```python
from build123d import *

# Parameters (mm, degrees)
F0_R     = 25
F1_DEPTH = 75
F0_R_2   = 37.5
F2_DEPTH = 50
F3_R     = 18
F4_DEPTH = 37.501
F5_R     = 25
F6_DEPTH = 37.5010001
F7_R     = 25
F8_DEPTH = 800


with BuildPart() as f1:
    # F0 (on Top) → F1 (new body, symmetric)
    with BuildSketch(Plane.XY):
        Circle(F0_R)
    extrude(amount=F1_DEPTH, both=True)

    # F0 (on Top) → F2 (join, symmetric)
    with BuildSketch(Plane.XY):
        Circle(F0_R_2)
        Circle(F0_R, mode=Mode.SUBTRACT)
    extrude(amount=F2_DEPTH, both=True)

    # F3 (on Right) → F4 (cut, through all)
    with BuildSketch(Plane.YZ):
        Circle(F3_R)
    extrude(amount=-F4_DEPTH, mode=Mode.SUBTRACT)

    # F5 (on Right) → F6 (cut, through all)
    with BuildSketch(Plane.YZ):
        Circle(F5_R)
    extrude(amount=F6_DEPTH, mode=Mode.SUBTRACT)

    # F7 (on face) → F8 (join)
    with BuildSketch(Plane.XY.offset(75)):
        Circle(F7_R)
    extrude(amount=F8_DEPTH)


solid = f1.part
```
The model under review builds one solid part; all positions refer to its coordinate system, in mm. A direction names the side the tool comes from. Round coordinates to 2 decimals unless told otherwise and drop trailing zeros. Loops run counter-clockwise (first coordinate to the right, second up) from the corner with the lowest first, then second, coordinate; pieces in that order, holes last. Notation, with made-up numbers: (88, 72.25) -> (106, 72.25) arc R20 cw to (106, 111.25) -> close; hole circle Ø6 at (3.25, 80). An arc over 180 degrees is marked (long way). Answer as a JSON object with one key per item and string values. Group by question number.
1) For line 1 (Z direction, x = 23, y = 0); line 2 (Z direction, x = -10.5, y = 0); line 3 (Y direction, x = 5.5, z = 13.5), list the stretches that pass through material, from the lowest coordinate up. Write a range as [from, to].
2) We need section D-D on z = 463.5. Write out the cut boundary in (x, y), then the cut area to 3 significant figures.
3) We need section A-A on y = 0. Write out the cut boundary in (x, z), then the cut area to 3 significant figures.
4) We need section C-C on z = 0. Write out the cut boundary in (x, y), then the cut area to 3 significant figures.
5) We need section B-B on x = -8. Write out the cut boundary in (y, z).
6) For faces 5 (the face through (23.846, 7.509, -62.325)), 6 (the face through (18, -20, -15)), 7 (the face through (0, 0, 875)), list the 3-axis set-ups (+Z, -Z, +X, -X, +Y, -Y) from which the entire face can be reached by the end or side of a thin tool; tool diameter is ignored.
7) Mouldability with a two-part tool opening along Z and no side actions: class faces 1 (the face through (24, -8, 50)), 2 (the face through (-18.488, 17.169, 5.407)), 3 (the face through (0, 0, -75)), 4 (the face through (0, 11, -16)) as released by +Z, released by -Z, zero draft, split by the parting line, or undercut.
8) For pin 1 Ø3 at (x, z) = (-5.5, 257) entering from +Y; pin 2 Ø2 at (x, z) = (-5.5, 300.5) entering from +Y; pin 3 Ø12 at (x, y) = (29.5, 23) entering from -Z, all flat-tipped, find the tip position at first contact; note any pin that passes through.
Result set:
{
 "1": {"line 1": "[-75, -25], [25, 875]", "line 2": "[-75, -18], [18, 875]", "line 3": "[-37.09, -21.04], [21.04, 37.09]"},
 "2": {"outline": "circle Ø50 at (0, 0)", "area": "1,960 mm²"},
 "3": {"outline": "(-37.5, -50) -> (-25, -50) -> (-25, -75) -> (25, -75) -> (25, -50) -> (37.5, -50) -> (37.5, -25) -> (0, -25) -> (0, -18) -> (-37.5, -18) -> close; (-37.5, 18) -> (0, 18) -> (0, 25) -> (37.5, 25) -> (37.5, 50) -> (25, 50) -> (25, 875) -> (-25, 875) -> (-25, 50) -> (-37.5, 50) -> close", "area": "46,800 mm²"},
 "4": {"outline": "(-32.9, -18) arc R37.5 ccw to (27.95, -25) -> (0, -25) -> (0, -18) -> close; (-32.9, 18) -> (0, 18) -> (0, 25) -> (27.95, 25) arc R37.5 ccw to start", "area": "1,400 mm²"},
 "5": {"outline": "(-36.64, -50) -> (-23.69, -50) -> (-23.69, -75) -> (23.69, -75) -> (23.69, -50) -> (36.64, -50) -> (36.64, 50) -> (23.69, 50) -> (23.69, 875) -> (-23.69, 875) -> (-23.69, 50) -> (-36.64, 50) -> close; hole circle Ø36 at (0, 0)"},
 "6": {"face 5": "-Z", "face 6": "+X", "face 7": "+Z, +X, -X, +Y, -Y"},
 "7": {"face 1": "released by +Z", "face 2": "undercut", "face 3": "released by -Z", "face 4": "undercut"},
 "8": {"pin 1": "y = 24.68", "pin 2": "y = 24.59", "pin 3": "z = -50"}
}
